For this review, take the finished solid that the model builds, in its own axes (mm). Face numbers are marked on the shaded views. A direction names the side the tool comes from. Round coordinates to 2 decimals unless told otherwise and drop trailing zeros. Write each loop counter-clockwise with the first axis right and the second up, starting at its lowest first coordinate (ties: lowest second). Pieces come first, ordered by that corner, then holes. Notation, with made-up numbers: M 34.5,39 L 52.5,39 A17 cw 52.5,70 Z; hole C -24.75,55.5 d3. An arc over 180 degrees is marked long. Write each question's results on one line, items separated by ' | '. Start each with the question number.
```python
from build123d import *

# Parameters (mm, degrees)
F0_W        = 70
F0_H        = 50
F0_W_2      = 40
F0_H_2      = 20
F2_DEPTH    = 10
F1_W        = 70
F1_H        = 50
F1_W_2      = 40
F1_H_2      = 20
F2_FACE_W   = 70
F2_FACE_H   = 50
F2_FACE_W_2 = 40
F2_FACE_H_2 = 20
F3_DEPTH    = 10
F4_DEPTH    = 10


with BuildPart() as f2:
    # F0 (on Front) → F2 (new body)
    with BuildSketch(Plane.XZ):
        with Locations((35, 25)):
            Rectangle(F0_W, F0_H)
        with Locations((30, 20)):
            Rectangle(F0_W_2, F0_H_2, mode=Mode.SUBTRACT)
    extrude(amount=F2_DEPTH)

    # F1 (on face) + F2_face (on face) → F3 (join)
    with BuildSketch(Plane.XZ):
        with Locations((35, 25)):
            Rectangle(F1_W, F1_H)
        with Locations((30, 20)):
            Rectangle(F1_W_2, F1_H_2, mode=Mode.SUBTRACT)
    with BuildSketch(Plane(origin=(36.4814814815, -10, 26.4814814815), x_dir=(1, 0, 0), z_dir=(0, -1, 0))):
        with Locations((-1.4814814815, -1.4814814815)):
            Rectangle(F2_FACE_W, F2_FACE_H)
        with Locations((-6.4814814815, -6.4814814815)):
            Rectangle(F2_FACE_W_2, F2_FACE_H_2, mode=Mode.SUBTRACT)
    extrude(amount=F3_DEPTH)

    # F4 (add): faces of the model
    f4_faces = [f2.faces().sort_by_distance(p)[0] for p in [
        (35, 0, 49.1397674733),
        (35, -20, 49.1397674733),
    ]]
    extrude(f4_faces, amount=F4_DEPTH, dir=(0, 1, 0))


solid = f2.part
```
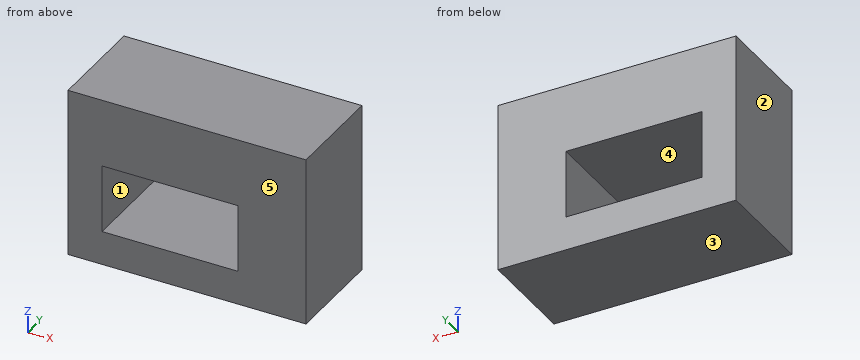
Item 1: We need section B-B on x = 46.5. State the section outline as (y, z) points, then the cut area to 3 significant figures.
Item 2: For the marked faces 4 and 5, list the 3-axis set-ups (+Z, -Z, +X, -X, +Y, -Y) from which the entire face can be reached by the end or side of a thin tool; tool diameter is ignored.
Item 3: Insertion check: P1, Ø5, axis at y = 1.5, z = 10.5, coming from the -X side. The pin has a flat end and moves straight along its axis. Give the tip position at first contact, or say it passes through.
Item 4: For probe 1 along X at (y, z) = (-1.25, 12); probe 2 along Z at (x, y) = (22.5, -5.5), list the stretches that pass through material, from the lowest coordinate up.
Item 5: Mouldability with a two-part tool opening along X and no side actions: class the marked faces 1, 2 and 3 as pulls with the +X half, pulls with the -X half, needs draft (parallel to the pull), parting line crosses it, or undercut.
Item 6: We need section A-A on z = 15. State the section outline as (x, y) points.
Item 7: We need section C-C on y = 5. State the section outline as (x, z) points.
Numbers:
1) outline: M -20,0 L 10,0 L 10,10 L -20,10 Z; M -20,30 L 10,30 L 10,50 L -20,50 Z | area: 900 mm^2
2) face 4: +Y, -Y | face 5: +Z, -Z, +X, -X, -Y
3) P1: stops at x = 0
4) probe 1: x = 0 to 10, 50 to 70 | probe 2: z = 0 to 10, 30 to 50
5) face 1: undercut | face 2: pulls with the -X half | face 3: needs draft
6) outline: M 0,-20 L 10,-20 L 10,10 L 0,10 Z; M 50,-20 L 70,-20 L 70,10 L 50,10 Z
7) outline: M 0,0 L 70,0 L 70,50 L 0,50 Z; hole M 10,10 L 50,10 L 50,30 L 10,30 Z
